```python
from build123d import *

# Parameters (mm, degrees)
SKETCH1_W               = 18
SKETCH1_H               = 20
BOSS_EXTRUDE1_DEPTH     = 60
SKETCH1_3_W             = 18
SKETCH1_3_H             = 20
CUT_EXTRUDE1_DEPTH      = 50
CUT_EXTRUDE3_DEPTH      = 28
CUT_EXTRUDE3_DEPTH_BACK = 70
SKETCH4_R               = 2
CUT_EXTRUDE4_DEPTH      = 57
CUT_EXTRUDE4_DEPTH_BACK = 57
SKETCH5_R               = 3
CHAMFER1_SIZE           = 10
CHAMFER1_SIZE2          = 27.474774195


with BuildPart() as part:
    # Sketch1 → Boss-Extrude1 (new body)
    with BuildSketch(Plane(origin=(0, 0, 0), x_dir=(1, 0, 0), z_dir=(0, 1, 0))):
        with Locations((0, -10)):
            Rectangle(SKETCH1_W, SKETCH1_H)
        Polygon((9, 0), (9, -20), (20, -20), (20, 20), (-20, 20), (-20, -20), (-9, -20), (-9, 0), align=None)
    extrude(amount=-BOSS_EXTRUDE1_DEPTH)

    # Sketch1_3 → Cut-Extrude1 (cut)
    with BuildSketch(Plane(origin=(0, 0, 0), x_dir=(1, 0, 0), z_dir=(0, 1, 0))):
        with Locations((0, -10)):
            Rectangle(SKETCH1_3_W, SKETCH1_3_H)
    extrude(amount=-CUT_EXTRUDE1_DEPTH, mode=Mode.SUBTRACT)

    # Sketch4 → Cut-Extrude3 (cut, two sides: drawn at the far end of the back side and taken through both)
    with BuildSketch(Plane(origin=(0, 0, 0), x_dir=(1, 0, 0), z_dir=(0, 1, 0)).offset(-CUT_EXTRUDE3_DEPTH_BACK)):
        with Locations(Location((-16, 16, 0), (0, 0, 270))):
            Circle(SKETCH4_R)
        with Locations(Location((16, 16, 0), (0, 0, 270))):
            Circle(SKETCH4_R)
        with Locations(Location((16, -0.977001598, 0), (0, 0, 270))):
            Circle(SKETCH4_R)
        with Locations(Location((-16, -0.977001598, 0), (0, 0, 270))):
            Circle(SKETCH4_R)
    extrude(amount=CUT_EXTRUDE3_DEPTH + CUT_EXTRUDE3_DEPTH_BACK, mode=Mode.SUBTRACT)

    # Sketch5 → Cut-Extrude4 (cut, two sides: drawn at the far end of the back side and taken through both)
    with BuildSketch(Plane.ZY.offset(-9).offset(-CUT_EXTRUDE4_DEPTH_BACK)):
        with Locations(Location((12.148726145, -25, 0), (0, 0, 180))):
            Circle(SKETCH5_R)
    extrude(amount=CUT_EXTRUDE4_DEPTH + CUT_EXTRUDE4_DEPTH_BACK, mode=Mode.SUBTRACT)

    # Chamfer1
    chamfer1_edges = [part.edges().sort_by_distance(p)[0] for p in [
        (-14.5, 0, 20),
        (14.5, 0, 20),
    ]]
    chamfer1_side = [part.faces().sort_by_distance(p)[0] for p in [
        (0, 0, -2.708529358),
    ]]
    chamfer(chamfer1_edges, length=CHAMFER1_SIZE, length2=CHAMFER1_SIZE2, reference=chamfer1_side[0])


solid = part.part
```
For this review, take the finished solid that the model builds, in its own axes (mm). A direction names the side the tool comes from. Coordinates: 2 decimals unless noted, no trailing zeros. Order: outer loops, then holes, each group sorted by start corner. A loop starts at its lowest first (then second) coordinate and runs counter-clockwise, first axis right, second up. Notation, with made-up numbers: (-3.5, -7) - (0.5, -7) arc R19 ccw to (0.5, 13) - close; hole circle Ø8 at (69, 5.25). An arc over 180 degrees is marked (long way). Answer as a JSON object with one key per item and string values. Group by question number.
1. The part is to be moulded in two halves that separate along X. For faces 1 (the flat face through (0, -60, 0)), 2 (the flat face through (20, -30, 0)), 3 (the flat face through (0, -25, 0)), say which applies: pulls with the +X half, pulls with the -X half, needs draft (parallel to the pull), parting line crosses it, or undercut.
2. We need section A-A on x = 16. State the section outline as (y, z) points, then the cut area to 3 significant figures.
3. For probe 1 along X at (y, z) = (-14.5, -16); probe 2 along X at (y, z) = (-28, 4); probe 3 along Z at (x, y) = (-17, -53.5), list the stretches that pass through material, from the lowest coordinate up.
4. We need section B-B on y = -25. State the section outline as (x, z) points, then the cut area to 3 significant figures.
5. We need section D-D on y = -41. State the section outline as (x, z) points.
6. For faces 4 (the flat face through (-9, -25, 8)), 5 (the cylindrical face through (-14, -30, -16)), list the 3-axis set-ups (+Z, -Z, +X, -X, +Y, -Y) from which the entire face can be reached by the end or side of a thin tool; tool diameter is ignored.
7. Clearance check with flat-ended pins moving along their axes: P1, Ø5, axis at x = -16, z = -16, coming from the -Y side; P2, Ø5, axis at y = -25, z = 12.15, coming from the +X side; P3, Ø5, axis at x = 4.5, z = 8, coming from the +Y side. State where each tip first meets the part, or that it passes through.
8. We need section C-C on z = -16. State the section outline as (x, y) points, then the cut area to 3 significant figures.
Final values:
{
 "1": {"face 1": "needs draft", "face 2": "pulls with the +X half", "face 3": "undercut"},
 "2": {"outline": "(-60, -20) - (0, -20) - (0, -18) - (-60, -18) - close; (-60, -14) - (0, -14) - (0, -1.02) - (-60, -1.02) - close; (-60, 2.98) - (0, 2.98) - (0, 10) - (-27.47, 20) - (-60, 20) - close; hole circle Ø6 at (-25, 12.15)", "area": "1,750 mm²"},
 "3": {"probe 1": "-20 to -18, -14 to 14, 18 to 20", "probe 2": "-20 to -9, 9 to 20", "probe 3": "-20 to -17.73, -14.27 to -0.76, 2.71 to 20"},
 "4": {"outline": "(-20, -20) - (20, -20) - (20, 9.15) - (9, 9.15) - (9, 0) - (-9, 0) - (-9, 9.15) - (-20, 9.15) - close; (-20, 15.15) - (-9, 15.15) - (-9, 19.1) - (-20, 19.1) - close; (9, 15.15) - (20, 15.15) - (20, 19.1) - (9, 19.1) - close; hole circle Ø4 at (-16, -16); hole circle Ø4 at (-16, 0.98); hole circle Ø4 at (16, -16); hole circle Ø4 at (16, 0.98)", "area": "1,040 mm²"},
 "5": {"outline": "(-20, -20) - (20, -20) - (20, 20) - (9, 20) - (9, 0) - (-9, 0) - (-9, 20) - (-20, 20) - close; hole circle Ø4 at (-16, -16); hole circle Ø4 at (-16, 0.98); hole circle Ø4 at (16, -16); hole circle Ø4 at (16, 0.98)"},
 "6": {"face 4": "+Z, +Y", "face 5": "+Y, -Y"},
 "7": {"P1": "y = -60", "P2": "through", "P3": "y = -50"},
 "8": {"outline": "(-20, -60) - (-18, -60) - (-18, 0) - (-20, 0) - close; (-14, -60) - (14, -60) - (14, 0) - (-14, 0) - close; (18, -60) - (20, -60) - (20, 0) - (18, 0) - close", "area": "1,920 mm²"}
}
